```python
from build123d import *

# Parameters (mm, degrees)
F0_W     = 30
F0_H     = 30
F0_R     = 5
F1_DEPTH = 7
F0_R_2   = 4
F2_DEPTH = 16.5
F3_DEPTH = 23.5
F5_D     = 5


with BuildPart() as f1:
    # F0 (on Top) → F1 (new body)
    with BuildSketch(Plane.XY):
        Rectangle(F0_W, F0_H)
        Circle(F0_R, mode=Mode.SUBTRACT)
    extrude(amount=F1_DEPTH)

    # F0 (on Top) → F2 (join)
    with BuildSketch(Plane.XY):
        Circle(F0_R)
        Circle(F0_R_2, mode=Mode.SUBTRACT)
    extrude(amount=F2_DEPTH)

    # F0 (on Top) → F3 (join)
    with BuildSketch(Plane.XY):
        Circle(F0_R_2)
    extrude(amount=F3_DEPTH)

    # F5 (through all)
    with Locations(Plane.XY.offset(7)):
        with Locations((8.5, 8.5), (-8.5, 8.5), (-8.5, -8.5), (8.5, -8.5)):
            Hole(F5_D / 2)


solid = f1.part
```
Work out the finished part from the listing and answer in its coordinate system (mm). A direction names the side the tool comes from. Round coordinates to 2 decimals unless told otherwise and drop trailing zeros. Order: outer loops, then holes, each group sorted by start corner. A loop starts at its lowest first (then second) coordinate and runs counter-clockwise, first axis right, second up.
Q1. Find the intervals of material crossed by line 1 along Y through (x, z) = (8.5, 2); line 2 along Z through (x, y) = (-3, -5); line 3 along Z through (x, y) = (-2.25, 4), in increasing order.
Solution:
line 1: y = -15 to -11, -6 to 6, 11 to 15
line 2: z = 0 to 7
line 3: z = 0 to 16.5
Q2. Given pin 1 Ø3 at (x, y) = (4.5, 6) entering from -Z; pin 2 Ø6 at (x, y) = (8.5, -10) entering from +Z; pin 3 Ø3 at (x, z) = (3, 13.5) entering from +Y, each flat-ended and moving along its own axis, determine where each tip first touches the part or whether it passes through.
Solution:
pin 1: stops at z = 0
pin 2: stops at z = 7
pin 3: stops at y = 4.77
Q3. A tool of negligible diameter and unlimited length cuts with its end or side. For faces 1 (the cylindrical face through (-0.867, -3.905, 19.951)), 2 (the cylindrical face through (-7.96, -10.94, 3.45)), from which of +Z, -Z, +X, -X, +Y, -Y can it reach the whole face along a straight path? Write none if from no direction.
Solution:
face 1: +Z
face 2: +Z, -Z
Q4. The mould has two halves that part along X. Classify faces 3 (the flat face through (0, 15, 3)), 4 (the cylindrical face through (9.04, 6.06, 3.45)), 5 (the cylindrical face through (-1.08, -4.88, 11.68)): pulls with the +X half, pulls with the -X half, needs draft (parallel to the pull), parting line crosses it, or undercut.
Solution:
face 3: needs draft
face 4: undercut
face 5: parting line crosses it
Q5. A cutting plane is placed at C-C, the plane y = 0. Determine the outline of the cut face in (x, z).
Solution:
outline: (-15, 0) - (15, 0) - (15, 7) - (5, 7) - (5, 16.5) - (4, 16.5) - (4, 23.5) - (-4, 23.5) - (-4, 16.5) - (-5, 16.5) - (-5, 7) - (-15, 7) - close
Q6. A cutting plane is placed at A-A, the plane y = -8.5. Determine the outline of the cut face in (x, z).
Solution:
outline: (-15, 0) - (-11, 0) - (-11, 7) - (-15, 7) - close; (-6, 0) - (6, 0) - (6, 7) - (-6, 7) - close; (11, 0) - (15, 0) - (15, 7) - (11, 7) - close
